Geometry: final body of the model. Coordinates: model frame, mm. Face numbers are marked on the shaded views. A direction names the side the tool comes from. Coordinates: 2 decimals unless noted, no trailing zeros. Write each loop counter-clockwise with the first axis right and the second up, starting at its lowest first coordinate (ties: lowest second). Pieces come first, ordered by that corner, then holes. Notation, with made-up numbers: (31.25, 38) -> (76.25, 38) arc R11 cw to (76.25, 56) -> close; hole circle Ø10 at (75.25, -5.5). An arc over 180 degrees is marked (long way). One line per item, written item: value. Start each with the question number.
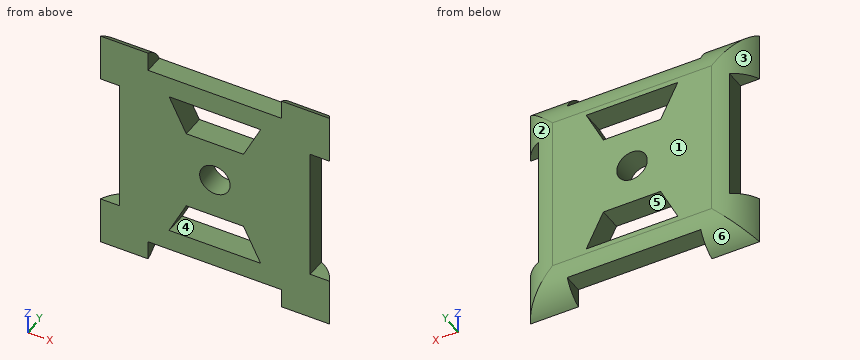
from build123d import *

# Parameters (mm, degrees)
SKETCH_1_W          = 20
SKETCH_1_H          = 20
EXTRUDE_1_DEPTH     = 2
CUT_EXTRUDE_1_DEPTH = 17.713614462
SCALE_1_SCALE       = 0.6
SKETCH_5_W          = 7
SKETCH_5_H          = 1
SKETCH_5_W_2        = 1
SKETCH_5_H_2        = 7
CUT_EXTRUDE_2_DEPTH = 12.05686647
FILLET_1_R          = 2
SKETCH_6_R          = 0.8
CUT_EXTRUDE_3_DEPTH = 12.05686647


with BuildPart() as part:
    # 草图1 → 凸台-拉伸1 (new body)
    with BuildSketch(Plane(origin=(0, 0, 0), x_dir=(1, 0, 0), z_dir=(0, 1, 0))):
        with Locations((-0.331632653, 2.984693878)):
            Rectangle(SKETCH_1_W, SKETCH_1_H)
    extrude(amount=EXTRUDE_1_DEPTH)

    # 草图2 → 切除-拉伸1 (cut, through all)
    with BuildSketch(Plane(origin=(0, 2, 0), x_dir=(1, 0, 0), z_dir=(0, 1, 0))):
        Polygon((-4.331632653, 9.484693878), (3.668367347, 9.484693878), (2.168367347, 6.484693878), (-2.831632653, 6.484693878), align=None)
        Polygon((3.668367347, -3.515306122), (2.168367347, -0.515306122), (-2.831632653, -0.515306122), (-4.331632653, -3.515306122), align=None)
    extrude(amount=-CUT_EXTRUDE_1_DEPTH, mode=Mode.SUBTRACT)


with BuildPart() as part_1:
    # 缩放比例1: scaled about (-0.331632653, 1, -2.984693878)
    add(part.part.scale(SCALE_1_SCALE).moved(Location((-0.132653061, 0.4, -1.193877551))))

    # 草图5 → 切除-拉伸2 (cut, through all)
    with BuildSketch(Plane(origin=(0, 1.6, 0), x_dir=(1, 0, 0), z_dir=(0, 1, 0))):
        with Locations((-0.331632653, -2.515306122)):
            Rectangle(SKETCH_5_W, SKETCH_5_H)
        with Locations((-5.831632653, 2.984693878)):
            Rectangle(SKETCH_5_W_2, SKETCH_5_H_2)
        with Locations((-0.331632653, 8.484693878)):
            Rectangle(SKETCH_5_W, SKETCH_5_H)
        with Locations((5.168367347, 2.984693878)):
            Rectangle(SKETCH_5_W_2, SKETCH_5_H_2)
    extrude(amount=-CUT_EXTRUDE_2_DEPTH, mode=Mode.SUBTRACT)

    # 圆角1
    # the kernel refuses this fillet: 2 mm, written as the material it takes off along each edge
    with BuildSketch(Plane(origin=(5.668367347, 1.6, -4.067269573), x_dir=(-1, 0, 0), z_dir=(0, 0, 1)), Plane(origin=(-1.414208348, 1.6, -8.984693878), x_dir=(0, 0, 1), z_dir=(1, 0, 0)), Plane(origin=(-6.331632653, 1.6, -1.902118183), x_dir=(1, 0, 0), z_dir=(0, 0, -1)), Plane(origin=(-6.331632653, 1.6, 7.597881817), x_dir=(1, 0, 0), z_dir=(0, 0, -1)), Plane(origin=(10.250943042, 1.6, 3.015306122), x_dir=(0, 0, -1), z_dir=(-1, 0, 0)), Plane(origin=(5.668367347, 1.6, -13.567269573), x_dir=(-1, 0, 0), z_dir=(0, 0, 1)), Plane(origin=(0.750943042, 1.6, 3.015306122), x_dir=(0, 0, -1), z_dir=(-1, 0, 0))) as fillet_1_piece_1:
        with BuildLine():
            CenterArc((1.833030278, 2), FILLET_1_R, 203.578178478, 66.421821522)
            Line((0, 1.2), (0, 0))
            Line((0, 0), (1.833030278, 0))
        make_face()
    extrude(amount=11.66515139, mode=Mode.SUBTRACT)
    with BuildSketch(Plane(origin=(-10.914208348, 1.6, -8.984693878), x_dir=(0, -1, 0), z_dir=(1, 0, 0))) as fillet_1_piece_2:
        with BuildLine():
            CenterArc((2, -1.833030278), FILLET_1_R, 113.578178478, 66.421821522)
            Line((0, -1.833030278), (0, 0))
            Line((0, 0), (1.2, 0))
        make_face()
    extrude(amount=11.66515139, mode=Mode.SUBTRACT)

    # 草图6 → 切除-拉伸3 (cut, through all)
    with BuildSketch(Plane.XZ.offset(-0.4)):
        with Locations(Location((-0.331632653, -2.984693878, 0), (0, 0, 270))):
            Circle(SKETCH_6_R)
    extrude(amount=-CUT_EXTRUDE_3_DEPTH, mode=Mode.SUBTRACT)


solid = part_1.part
Q1. Cut plane C-C on z = 0. Output: boundary loops of the cut face in (x, y), and give its area (3 significant figures).
Q2. Line query: L1, parallel to Z at x = -1.75, y = 0.9; L2, parallel to Z at x = 2.5, y = 0.95; L3, parallel to X at y = 0.7, z = -5. Output: solid intervals per line, ascending. Write a range as from..to.
Q3. Access query for the marked faces 5 and 6. Directions: +Z, -Z, +X, -X, +Y, -Y. A direction counts if a zero-diameter tool reaches every point of the face in a straight line with its end or side. Return the directions, or none.
Q4. Draft query along X for the marked faces 1, 2, 3 and 4. Return one class per face: pulls with the +X half, pulls with the -X half, needs draft (parallel to the pull), parting line crosses it, or undercut.
Q5. First-contact query: P1, Ø0.6, axis at x = 0, y = 1, coming from the +Z side; P2, Ø0.5, axis at y = 1, z = -8.5, coming from the +X side. Flat tips, straight axial feed; report the tip coordinate or a pass-through.
Q6. Cut plane A-A on x = 1.5. Output: boundary loops of the cut face in (y, z).
Q7. Cut plane B-B on y = 0.65. Count the separate pieces of the cut face and the enclosed holes in it, and give its area (3 significant figures).
Q8. Cut plane D-D on x = -0.5. Output: boundary loops of the cut face in (y, z), and give its area (3 significant figures).
Solution:
1. outline: (-5.33, 0.4) -> (-2.27, 0.4) -> (-2.27, 1.6) -> (-4.5, 1.6) arc R2 ccw to (-5.33, 1.42) -> close; (1.61, 0.4) -> (4.67, 0.4) -> (4.67, 1.42) arc R2 ccw to (3.84, 1.6) -> (1.61, 1.6) -> close
1. area: 7.24 mm²
2. L1: -7.98..-6.88, -5.08..-0.88, 0.92..2.02
2. L2: -7.98..2.02
2. L3: -5.33..4.67
3. face 5: +Y, -Y
3. face 6: -Z, +X, -X, +Y
4. face 1: needs draft
4. face 2: pulls with the +X half
4. face 3: pulls with the -X half
4. face 4: undercut
5. P1: z = 2.02
5. P2: x = 5.47
6. outline: (0.4, -7.98) -> (1.42, -7.98) arc R2 ccw to (1.6, -7.15) -> (1.6, -6.88) -> (0.4, -6.88) -> close; (0.4, -5.75) -> (1.6, -5.75) -> (1.6, -0.22) -> (0.4, -0.22) -> close; (0.4, 0.92) -> (1.6, 0.92) -> (1.6, 1.18) arc R2 ccw to (1.42, 2.02) -> (0.4, 2.02) -> close
7. separate pieces: 1
7. enclosed holes: 3
7. area: 97.4 mm²
8. outline: (0.4, -7.98) -> (1.42, -7.98) arc R2 ccw to (1.6, -7.15) -> (1.6, -6.88) -> (0.4, -6.88) -> close; (0.4, -5.08) -> (1.6, -5.08) -> (1.6, -3.77) -> (0.4, -3.77) -> close; (0.4, -2.2) -> (1.6, -2.2) -> (1.6, -0.88) -> (0.4, -0.88) -> close; (0.4, 0.92) -> (1.6, 0.92) -> (1.6, 1.18) arc R2 ccw to (1.42, 2.02) -> (0.4, 2.02) -> close
8. area: 5.70 mm²
